Autodesk Inventor part; units mm, degrees
ref_plane "РабПлоскость1" through (-18, 0, 0) normal (0, 0, 1) x (1, 0, 0)
ref_plane "YZ Plane" through (0, 0, 0) normal (1, 0, 0) x (0, 1, 0)
ref_plane "XZ Plane" through (0, 0, 0) normal (0, 1, 0) x (-1, 0, 0)
sketch "Эскиз1" plane through (0, 0, 0) normal (0, 1, 0) x (-1, 0, 0)
  line L0 (18, -35.15) -> (-18, -35.15)
  line L1 (-18, -35.15) -> (-18, 35.15)
  line L2 (-18, 35.15) -> (18, 35.15)
  line L3 (18, 35.15) -> (18, -35.15)
  line L4 (18, -35.15) -> (-18, 35.15) construction
  line L5 (-18, -35.15) -> (18, 35.15) construction
  line L6 (15.375, -30.85) -> (-15.375, -30.85) construction
  line L7 (-15.375, -30.85) -> (-15.375, 30.85) construction
  line L8 (-15.375, 30.85) -> (15.375, 30.85) construction
  line L9 (15.375, 30.85) -> (15.375, -30.85) construction
  line L10 (15.375, -30.85) -> (-15.375, 30.85) construction
  line L11 (-15.375, -30.85) -> (15.375, 30.85) construction
  circle A0 centre (15.375, -30.85) radius 1.75
  line L12 (0, 0) -> (0, -35.15) construction
  line L13 (18, 0) -> (-18, 0) construction
  line L14 (15.375, -30.85) -> (-15.375, 30.85) construction
  circle A1 centre (-15.375, -30.85) radius 1.75
  line L15 (-18, 0) -> (18, 0) construction
  circle A2 centre (15.375, 30.85) radius 1.75
  circle A3 centre (-15.375, 30.85) radius 1.75
  point P0 (0, 0)
  dimension "d0" = 36
  dimension "d1" = 70.3
  dimension "d2" = 30.75
  dimension "d3" = 61.7
  dimension "d4" = 3.5
extrude "Выдавливание1" add sketch "Эскиз1" along normal blind 1.5
sketch "Эскиз2" plane through (0, 1.5, 0) normal (0, 1, 0) x (1, 0, 0)
  circle A0 centre (0, 0) radius 15
  circle A1 centre (0, 0) radius 7.5
  dimension "d7" = 30
  dimension "d8" = 15
extrude "Выдавливание2" add sketch "Эскиз2" along normal blind 17
sketch "Эскиз4" plane through (0, 1.5, 0) normal (0, 1, 0) x (1, 0, 0)
  circle A0 centre (-5.5, -26.15) radius 5
  line L0 (-18, -35.15) -> (18, -35.15)
  circle A1 centre (5.5, -26.15) radius 5
  line L1 (-18, 35.15) -> (-18, -35.15)
  line L2 (-18, 35.15) -> (-18, -35.15) construction
  line L3 (-18, 0) -> (18, 0) construction
  line L4 (18, -35.15) -> (18, 35.15) construction
  circle A2 centre (-5.5, 21.65) radius 5
  circle A3 centre (5.5, 21.65) radius 5
  line L5 (18, 35.15) -> (-18, 35.15)
  point P0 (0, 0)
  dimension "d11" = 10
  dimension "d12" = 9
  dimension "d13" = 10
  dimension "d14" = 9
  dimension "d15" = 11
  dimension "d16" = 12.5
  dimension "d19" = 10
  dimension "d20" = 10
  dimension "d21" = 13.5
  dimension "d22" = 13.5
  dimension "d23" = 11
  dimension "d24" = 12.5
extrude "Выдавливание3" add sketch "Эскиз4" along normal blind 10.5
ref_plane "РабПлоскость1" through (-18, 0, 0) normal (0, 0, 1) x (1, 0, 0)
fillet "Сопряжение1" radius 3 2 edges at (-15, 18.5, 0) (-7.5, 18.5, 0)
properties part number "a1401220"
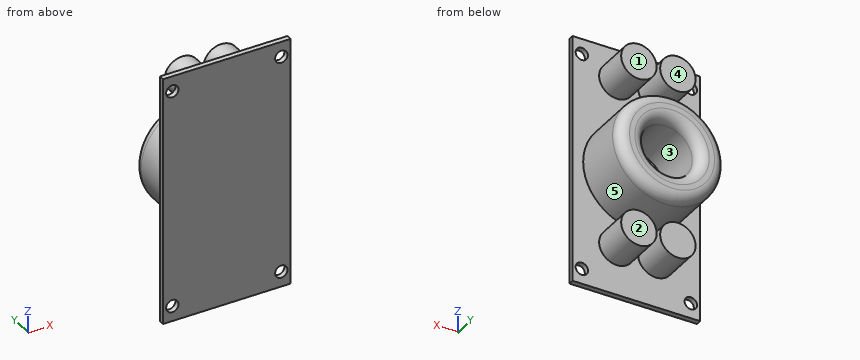
Design review of the part built by this model. Coordinates are the model's own, in mm. Face numbers are marked on the shaded views. A direction names the side the tool comes from. Coordinates: 2 decimals unless noted, no trailing zeros. Write each loop counter-clockwise with the first axis right and the second up, starting at its lowest first coordinate (ties: lowest second). Pieces come first, ordered by that corner, then holes. Notation, with made-up numbers: (51, -33) - (73, -33) arc R23 cw to (73, -7) - close; hole circle Ø1 at (80, 66.25). An arc over 180 degrees is marked (long way). Use one line per item in the form item = value.
Q1. Consider section C-C (z = -27.5). Write out the cut boundary in (x, y), plus the area to 3 significant figures.
Taken from the geometry:
outline = (-18, 0) - (18, 0) - (18, 1.5) - (-18, 1.5) - close
area = 54.0 mm^2
Q2. Consider section A-A (y = 6.25). Write out the cut boundary in (x, z), plus the area to 3 significant figures.
Taken from the geometry:
outline = circle Ø30 at (0, 0); circle Ø10 at (-5.5, -21.65); circle Ø10 at (-5.5, 26.15); circle Ø10 at (5.5, -21.65); circle Ø10 at (5.5, 26.15); hole circle Ø15 at (0, 0)
area = 844 mm^2
Q3. For probe 1 along X at (y, z) = (12, 0); probe 2 along Z at (x, y) = (4, 9.75); probe 3 along Z at (x, y) = (-3.5, 5), list the stretches that pass through material, from the lowest coordinate up.
Taken from the geometry:
probe_1 = -15 to -7.5, 7.5 to 15
probe_2 = -26.42 to -16.88, -14.46 to -6.34, 6.34 to 14.46, 21.38 to 30.92
probe_3 = -26.23 to -17.07, -14.59 to -6.63, 6.63 to 14.59, 21.57 to 30.73
Q4. The part is to be moulded in two halves that separate along Z. For the marked faces 4 and 5, say which applies: +Z half, -Z half, draft (parallel to the pull), parting line (faces both ways), or undercut.
Taken from the geometry:
face_4 = draft
face_5 = undercut
Q5. Consider section B-B (z = 26.15). Write out the cut boundary in (x, y), plus the area to 3 significant figures.
Taken from the geometry:
outline = (-18, 0) - (18, 0) - (18, 1.5) - (10.5, 1.5) - (10.5, 12) - (0.5, 12) - (0.5, 1.5) - (-0.5, 1.5) - (-0.5, 12) - (-10.5, 12) - (-10.5, 1.5) - (-18, 1.5) - close
area = 264 mm^2
Q6. Machinability: for the marked faces 1, 2 and 3, which of the approach directions +Z, -Z, +X, -X, +Y, -Y give a long, thin tool a straight path to every point of the face, cutting with its end or side? Answer none if there is none.
Taken from the geometry:
face_1 = +Z, +X, -X, +Y
face_2 = -Z, +X, -X, +Y
face_3 = +Y
Q7. Insertion check: pin 1 Ø12 at (x, z) = (0, 0) entering from +Y; pin 2 Ø8 at (x, z) = (7, 27.5) entering from +Y; pin 3 Ø5 at (y, z) = (15, 6.5) entering from -X; pin 4 Ø3 at (x, z) = (15.375, 30.85) entering from +Y. Each pin has a flat end and moves straight along its axis. Give the tip position at first contact, or say it passes through.
Taken from the geometry:
pin_1 = 1.5
pin_2 = 12
pin_3 = -14.46
pin_4 = through
